Geometry: final body of the model. Coordinates: model frame, mm. A direction names the side the tool comes from. Give positions to 0.01 mm unless a question says otherwise; leave off trailing zeros. Order: outer loops, then holes, each group sorted by start corner. A loop starts at its lowest first (then second) coordinate and runs counter-clockwise, first axis right, second up. Notation, with made-up numbers: (85.25, 86) -> (110.25, 86) arc R26 cw to (110.25, 119) -> close; hole circle Ø6 at (75.5, 46.5). An arc over 180 degrees is marked (long way). Write item = value, one per line.
```python
from build123d import *

# Parameters (mm, degrees)
F0_R     = 21.971
F0_R_2   = 15.621
F1_DEPTH = 6.35
F2_DEPTH = 19.05
F3_R     = 4.7625
F4_DEPTH = 19.051


with BuildPart() as f1:
    # F0 (on Top) → F1 (new body)
    with BuildSketch(Plane.XY):
        Circle(F0_R)
        Circle(F0_R_2, mode=Mode.SUBTRACT)
    extrude(amount=F1_DEPTH)

    # F0 (on Top) → F2 (join)
    with BuildSketch(Plane.XY):
        Circle(F0_R_2)
    extrude(amount=F2_DEPTH)

    # F3 (on face) → F4 (cut, through all)
    with BuildSketch(Plane.XY.offset(19.05)):
        Circle(F3_R)
    extrude(amount=-F4_DEPTH, mode=Mode.SUBTRACT)


solid = f1.part
```
1) Section query D-D (y = 11). Output: boundary loops of the cut face in (x, z), plus the area to 3 significant figures.
Check sheet entries:
outline = (-19.02, 0) -> (19.02, 0) -> (19.02, 6.35) -> (11.09, 6.35) -> (11.09, 19.05) -> (-11.09, 19.05) -> (-11.09, 6.35) -> (-19.02, 6.35) -> close
area = 523 mm²
2) Mould query, pull axis X, two halves, no side actions, for faces 1 (the face through (20.956, 6.599, 3.131)), 2 (the face through (-3.78, -2.9, 9.66)), 3 (the face through (5, 15, 6.35)). Classes: +X half, -X half, draft (parallel to the pull), parting line (faces both ways), or undercut.
Check sheet entries:
face_1 = parting line
face_2 = undercut
face_3 = draft
3) Section query C-C (z = 13.5). Output: boundary loops of the cut face in (x, y) (1 decimal), plus the area to 3 significant figures.
Check sheet entries:
outline = circle Ø31.2 at (0, 0); hole circle Ø9.5 at (0, 0)
area = 695 mm²
4) First-contact query: P1, Ø6, axis at x = -10, z = 6.5, coming from the -Y side; P2, Ø8, axis at x = 4, z = 17, coming from the -Y side; P3, Ø4, axis at x = 12.5, z = 17, coming from the -Y side. Flat tips, straight axial feed; report the tip coordinate or a pass-through.
Check sheet entries:
P1 = -20.82
P2 = -15.62
P3 = -11.57
5) Section query A-A (y = 0). Output: boundary loops of the cut face in (x, z).
Check sheet entries:
outline = (-21.97, 0) -> (-4.76, 0) -> (-4.76, 19.05) -> (-15.62, 19.05) -> (-15.62, 6.35) -> (-21.97, 6.35) -> close; (4.76, 0) -> (21.97, 0) -> (21.97, 6.35) -> (15.62, 6.35) -> (15.62, 19.05) -> (4.76, 19.05) -> close
6) Line query: line 1 (Y direction, x = 0, z = 12.25); line 2 (Z direction, x = 20.5, y = -4.5); line 3 (Y direction, x = -2, z = 3.25). Output: solid intervals per line, ascending. Write a range as from..to.
Check sheet entries:
line_1 = -15.62..-4.76, 4.76..15.62
line_2 = 0..6.35
line_3 = -21.88..-4.32, 4.32..21.88
7) Reachability of faces 4 (the face through (3, 4, 19.05)), 5 (the face through (-2.03, 15.49, 12.61)) from +Z, -Z, +X, -X, +Y, -Y: full face, straight path, thin tool, end or side. Return the list, or none.
Check sheet entries:
face_4 = +Z, +X, -X, +Y, -Y
face_5 = +Z
